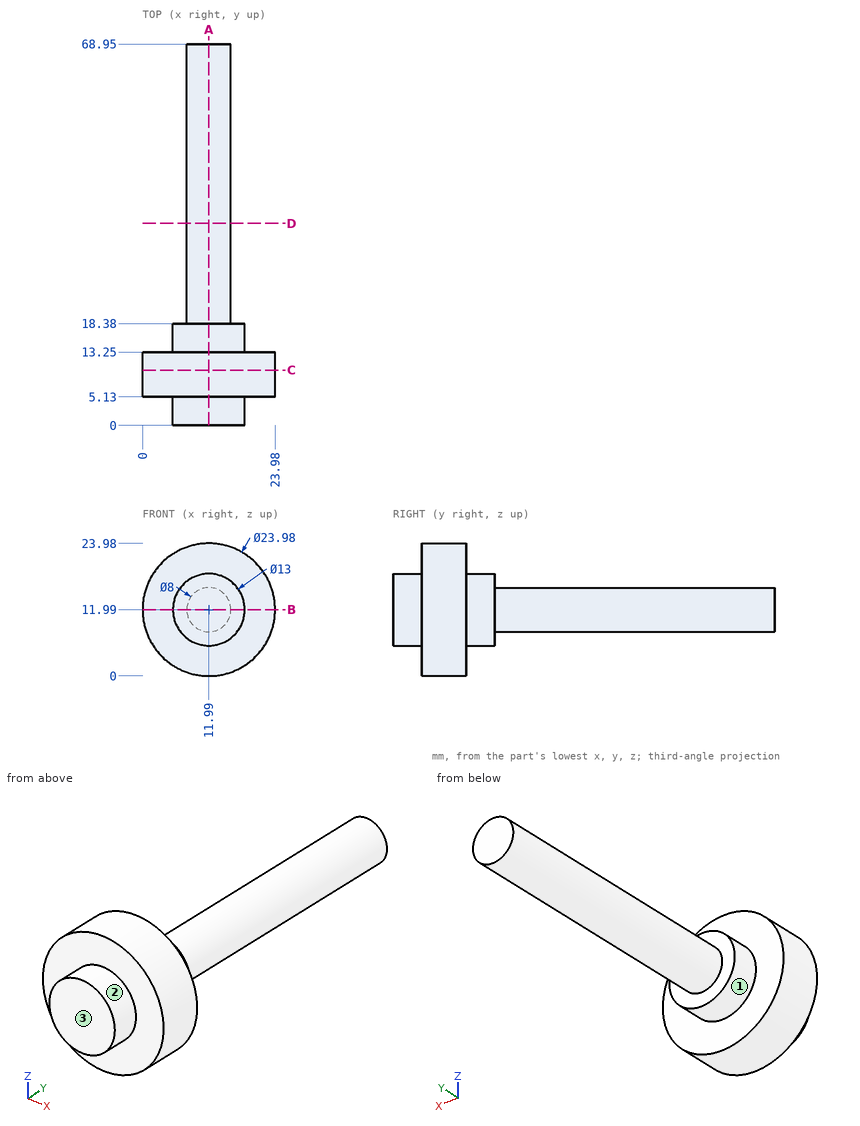
Print and shaded views of the part. All mm, measured from the part's lowest x, y and z. A direction names the side the tool comes from. Give positions to 0.01 mm unless a question says otherwise; leave off trailing zeros. Loops run counter-clockwise (first coordinate to the right, second up) from the corner with the lowest first, then second, coordinate; pieces in that order, holes last. Notation, with made-up numbers: (57.25, 79.25) -> (109.25, 79.25) arc R11 cw to (109.25, 92.25) -> close; hole circle Ø11 at (32.25, 19). An arc over 180 degrees is marked (long way). Answer in a Markdown table with one row per item.
Item 1: Tool access for the marked faces 1, 2 and 3: list every direction of +Z, -Z, +X, -X, +Y, -Y with a clear straight run to the whole face (end or side of a thin tool).
Findings below:
| item | result |
|---|---|
| face 1 | +Y |
| face 2 | -Y |
| face 3 | +Z, -Z, +X, -X, -Y |
Item 2: Probe line 1 along Y through (x, z) = (16.5, 3.75); line 2 along Y through (x, z) = (6.5, 14.25); line 3 along X through (y, z) = (6.5, 4.75). List the from-to ranges inside material, lowest first. Write a range as [from, to].
Findings below:
| item | result |
|---|---|
| line 1 | y = [5.13, 13.25] |
| line 2 | y = [0, 18.38] |
| line 3 | x = [2.43, 21.55] |
Item 3: Slice it at C-C on y = 10. Write the cut outline in (x, z), plus the area to 3 significant figures.
Findings below:
| item | result |
|---|---|
| outline | circle Ø23.98 at (11.99, 11.99) |
| area | 452 mm² |
Item 4: Slice it at D-D on y = 36.5. Write the cut outline in (x, z).
Findings below:
| item | result |
|---|---|
| outline | circle Ø8 at (11.99, 11.99) |
Item 5: Slice it at A-A on x = 11.99. Write the cut outline in (y, z), plus the area to 3 significant figures.
Findings below:
| item | result |
|---|---|
| outline | (0, 5.49) -> (5.13, 5.49) -> (5.13, 0) -> (13.25, 0) -> (13.25, 5.49) -> (18.38, 5.49) -> (18.38, 7.99) -> (68.95, 7.99) -> (68.95, 15.99) -> (18.38, 15.99) -> (18.38, 18.49) -> (13.25, 18.49) -> (13.25, 23.98) -> (5.13, 23.98) -> (5.13, 18.49) -> (0, 18.49) -> close |
| area | 733 mm² |
Item 6: Slice it at B-B on z = 11.99. Write the cut outline in (x, y).
Findings below:
| item | result |
|---|---|
| outline | (0, 5.13) -> (5.49, 5.13) -> (5.49, 0) -> (18.49, 0) -> (18.49, 5.13) -> (23.98, 5.13) -> (23.98, 13.25) -> (18.49, 13.25) -> (18.49, 18.38) -> (15.99, 18.38) -> (15.99, 68.95) -> (7.99, 68.95) -> (7.99, 18.38) -> (5.49, 18.38) -> (5.49, 13.25) -> (0, 13.25) -> close |
Item 7: Flat gauge pins, fed straight in: P1, Ø5, axis at x = 11.5, y = 52, coming from the +Z side; P2, Ø2, axis at x = 9.5, z = 20.5, coming from the -Y side; P3, Ø12, axis at x = 4, y = 30.5, coming from the -Z side; P4, Ø6, axis at x = 2.5, y = 29, coming from the +Z side. Where does each tip first touch, or does it go through?
Findings below:
| item | result |
|---|---|
| P1 | stops at z = 15.99 |
| P2 | stops at y = 5.13 |
| P3 | stops at z = 8.52 |
| P4 | passes through |
